The listing builds one solid part. Answer for the finished solid, in the listing's coordinates (mm). Face numbers are marked on the shaded views. A direction names the side the tool comes from. Round coordinates to 2 decimals unless told otherwise and drop trailing zeros. Write each loop counter-clockwise with the first axis right and the second up, starting at its lowest first coordinate (ties: lowest second). Pieces come first, ordered by that corner, then holes. Notation, with made-up numbers: (-25.5, 79.5) -> (12.5, 79.5) arc R3 cw to (12.5, 83.5) -> close; hole circle Ø4 at (3.25, 82). An arc over 180 degrees is marked (long way). Write each question's results on one line, items separated by ' | '. Start each with the question number.
```python
from build123d import *

# Parameters (mm, degrees)
SKETCH1_W          = 4.5
SKETCH1_H          = 10
BODY_SHAPE_DEPTH   = 2.5
SKETCH2_R          = 0.5
OFF_HOLE_DEPTH     = 1
SKETCH3_R          = 0.5
ON_HOLE_DEPTH      = 0.1
BOTTOM_FLAPS_DEPTH = 0.5
SKETCH4_R          = 0.3


with BuildPart() as part:
    # Sketch1 → Body Shape (new body)
    with BuildSketch(Plane(origin=(0, 0, 0), x_dir=(1, 0, 0), z_dir=(0, 1, 0))):
        with Locations((2.25, 5)):
            Rectangle(SKETCH1_W, SKETCH1_H)
    extrude(amount=BODY_SHAPE_DEPTH)

    # Sketch2 → Off Hole (cut)
    with BuildSketch(Plane.ZY):
        with Locations((-9.35, 1.25)):
            Circle(SKETCH2_R)
    extrude(amount=-OFF_HOLE_DEPTH, mode=Mode.SUBTRACT)

    # Sketch3 → On hole (cut)
    with BuildSketch(Plane.ZY):
        with Locations((-0.65, 1.25)):
            Circle(SKETCH3_R)
    extrude(amount=-ON_HOLE_DEPTH, mode=Mode.SUBTRACT)

    # Sketch8 → bottom flaps (add)
    with BuildSketch(Plane(origin=(4.5, 0, 0), x_dir=(0, 0, -1), z_dir=(1, 0, 0))):
        with BuildLine():
            Line((9.7, 0.123206048), (9.7, 2.376793952))
            ThreePointArc((9.7, 2.376793952), (9.575, 2.5), (9.45, 2.376793952))
            Line((9.45, 2.376793952), (9.45, 0.123206048))
            ThreePointArc((9.45, 0.123206048), (9.575, 0), (9.7, 0.123206048))
        make_face()
        with BuildLine():
            Line((0.3, 0.123206048), (0.3, 2.376793952))
            ThreePointArc((0.3, 2.376793952), (0.425, 2.5), (0.55, 2.376793952))
            Line((0.55, 2.376793952), (0.55, 0.123206048))
            ThreePointArc((0.55, 0.123206048), (0.425, 0), (0.3, 0.123206048))
        make_face()
    extrude(amount=BOTTOM_FLAPS_DEPTH)

    # pins: sweep along a path in Sketch9
    with BuildLine(Plane.XY.offset(-7.54)) as pins_path:
        Line((4.5, 1.25), (5, 1.25))
        ThreePointArc((5, 1.25), (5.353553391, 1.103553391), (5.5, 0.75))
        Line((5.5, 0.75), (5.5, -0.45))
    # Sketch4 → pins (sweep)
    with BuildSketch(Plane(origin=(4.5, 0, 0), x_dir=(0, 0, -1), z_dir=(1, 0, 0))):
        with Locations((7.54, 1.25)):
            Circle(SKETCH4_R)
        with Locations((5, 1.25)):
            Circle(SKETCH4_R)
        with Locations((2.46, 1.25)):
            Circle(SKETCH4_R)
    sweep(path=pins_path.line)


solid = part.part
```
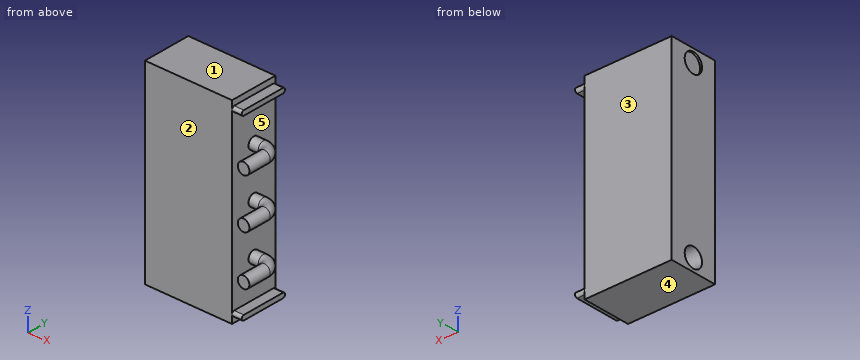
Q1. Determine the mould class of the marked faces 3, 4 and 5 for opening direction Z: pulls with the +Z half, pulls with the -Z half, needs draft (parallel to the pull), parting line crosses it, or undercut.
Q2. Find the intervals of material crossed by line 1 (X direction, y = 0.5, z = -5); line 2 (Y direction, x = 0.55, z = -9.35); line 3 (Z direction, x = 5.35, y = 0), in increasing order.
Q3. For the marked faces 1 and 2, determine the directions among +Z, -Z, +X, -X, +Y, -Y from which every point of the face is accessible in a straight line to the end or side of a thin tool.
Q4. The part is cut by section D-D, the plane x = 5.5. State how many separate pieces and enclosed holes the cut face has, then the cut area to 3 significant figures.
Q5. The part is cut by section A-A, the plane z = -9.35. Write down the section's boundary in (x, y).
Q6. The part is cut by section C-C, the plane y = 1.65. Write down the section's boundary in (x, z).
Q7. The part is cut by section B-B, the plane x = 0.55. Write down the section's boundary in (y, z), then the cut area to 3 significant figures.
Answers follow:
1) face 3: needs draft | face 4: pulls with the -Z half | face 5: undercut
2) line 1: 0 to 4.5, 5.2 to 5.8 | line 2: 0 to 0.75, 1.75 to 2.5 | line 3: -7.8 to -7.28, -5.26 to -4.74, -2.72 to -2.2
3) face 1: +Z, +X, -X, +Y, -Y | face 2: +Z, -Z, -X, -Y
4) separate pieces: 3 | enclosed holes: 0 | area: 3.12 mm^2
5) outline: (0, 0) -> (4.5, 0) -> (4.5, 2.5) -> (0, 2.5) -> (0, 1.75) -> (1, 1.75) -> (1, 0.75) -> (0, 0.75) -> close
6) outline: (0, -10) -> (4.5, -10) -> (4.5, -9.7) -> (5, -9.7) -> (5, -9.45) -> (4.5, -9.45) -> (4.5, -0.55) -> (5, -0.55) -> (5, -0.3) -> (4.5, -0.3) -> (4.5, 0) -> (0, 0) -> (0, -0.35) -> (0.1, -0.35) -> (0.1, -0.95) -> (0, -0.95) -> (0, -9.05) -> (1, -9.05) -> (1, -9.65) -> (0, -9.65) -> close
7) outline: (0, -10) -> (2.5, -10) -> (2.5, 0) -> (0, 0) -> close; hole circle Ø1 at (1.25, -9.35) | area: 24.2 mm^2
